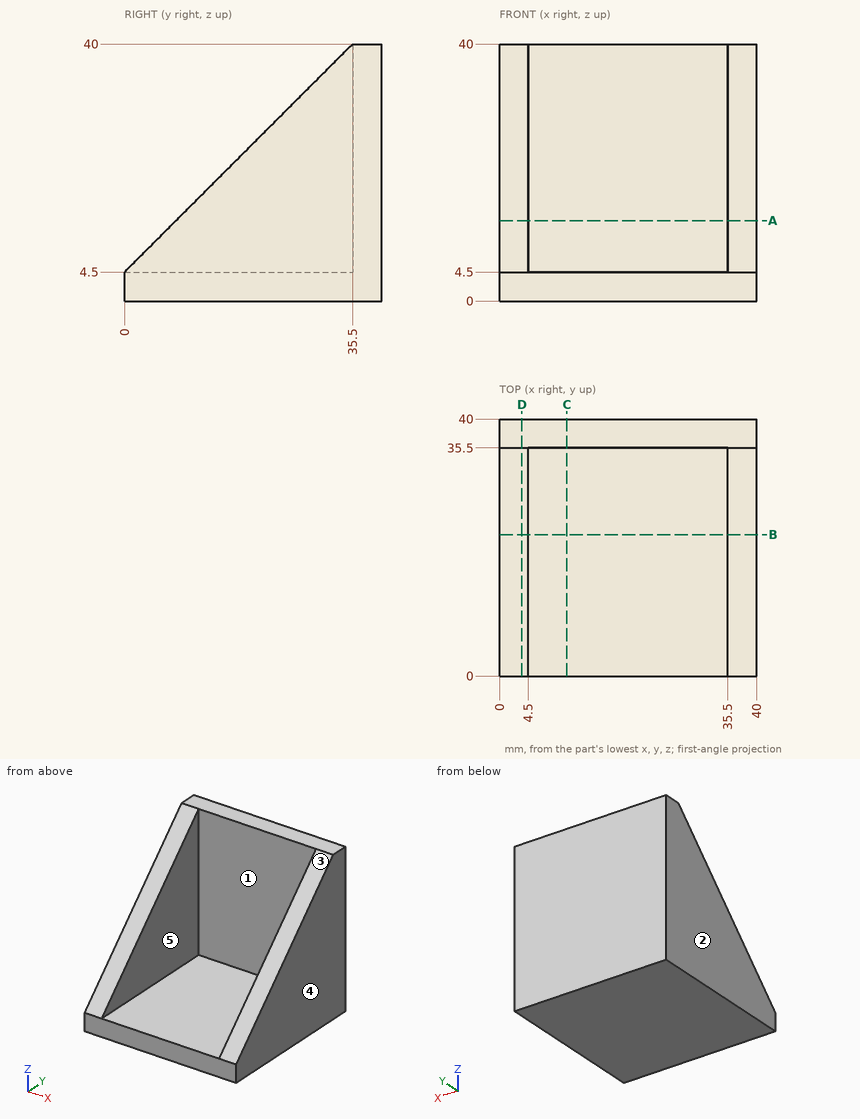
Job drawing, mm, ordinate dimensions from the low corner. One solid piece. A direction names the side the tool comes from. Give positions to 0.01 mm unless a question says otherwise; leave off trailing zeros. Write each loop counter-clockwise with the first axis right and the second up, starting at its lowest first coordinate (ties: lowest second). Pieces come first, ordered by that corner, then holes. Notation, with made-up numbers: (-21.5, 72) - (31.5, 72) arc R31 ccw to (31.5, 101) - close; hole circle Ø1 at (-3, 52.5). An arc over 180 degrees is marked (long way). Use one line per item in the form item = value. Start each with the question number.
1. Band-saw the part on C-C on x = 10.5. Write the cut outline in (y, z), plus the area to 3 significant figures.
2. Drop flat-ended pins along their axis: pin 1 Ø2 at (x, z) = (17, 22.5) entering from -Y; pin 2 Ø2 at (x, y) = (28.5, 20) entering from +Z; pin 3 Ø3 at (x, y) = (35.5, 10.5) entering from +Z. Give the stop position or say it passes through.
3. 3-axis set-ups, long thin cutter, end or side, ignore diameter. For the marked faces 1 and 2: which of +Z, -Z, +X, -X, +Y, -Y reach the whole face in a straight line?
4. Band-saw the part on A-A on z = 12.5. Write the cut outline in (x, y).
5. Probe line 1 (Z direction, x = 19, y = 24.5); line 2 (Y direction, x = 32.5, z = 26.5); line 3 (X direction, y = 34, z = 38). List the from-to ranges inside material, lowest first. Write a range as [from, to].
6. Band-saw the part on B-B on y = 22. Write the cut outline in (x, z).
7. Two-plate mould, pull along X, no slides. Class the marked faces 3, 4 and 5: released by +X, released by -X, zero draft, split by the parting line, or undercut.
8. Band-saw the part on D-D on x = 3.5. Write the cut outline in (y, z).
Conclusion:
q1.outline = (0, 0) - (40, 0) - (40, 40) - (35.5, 40) - (35.5, 4.5) - (0, 4.5) - close
q1.area = 340 mm²
q2.pin_1 = 35.5
q2.pin_2 = 4.5
q2.pin_3 = 16.5
q3.face_1 = +Z, -Y
q3.face_2 = +Z, -Z, -X, +Y, -Y
q4.outline = (0, 8) - (4.5, 8) - (4.5, 35.5) - (35.5, 35.5) - (35.5, 8) - (40, 8) - (40, 40) - (0, 40) - close
q5.line_1 = [0, 4.5]
q5.line_2 = [35.5, 40]
q5.line_3 = [0, 4.5], [35.5, 40]
q6.outline = (0, 0) - (40, 0) - (40, 26.5) - (35.5, 26.5) - (35.5, 4.5) - (4.5, 4.5) - (4.5, 26.5) - (0, 26.5) - close
q7.face_3 = zero draft
q7.face_4 = released by +X
q7.face_5 = undercut
q8.outline = (0, 0) - (40, 0) - (40, 40) - (35.5, 40) - (0, 4.5) - close
